For this review, use the dimensioned drawing (mm, ordinates from the lowest corner) and the shaded views. A direction names the side the tool comes from. Coordinates: 2 decimals unless noted, no trailing zeros. Write each loop counter-clockwise with the first axis right and the second up, starting at its lowest first coordinate (ties: lowest second). Pieces come first, ordered by that corner, then holes. Notation, with made-up numbers: (21.25, -8.5) -> (80.25, -8.5) arc R22 cw to (80.25, 2.5) -> close; hole circle Ø5 at (40, 12.5). An arc over 180 degrees is marked (long way). Return JSON: item names as keys, results as strings. Group by question number.
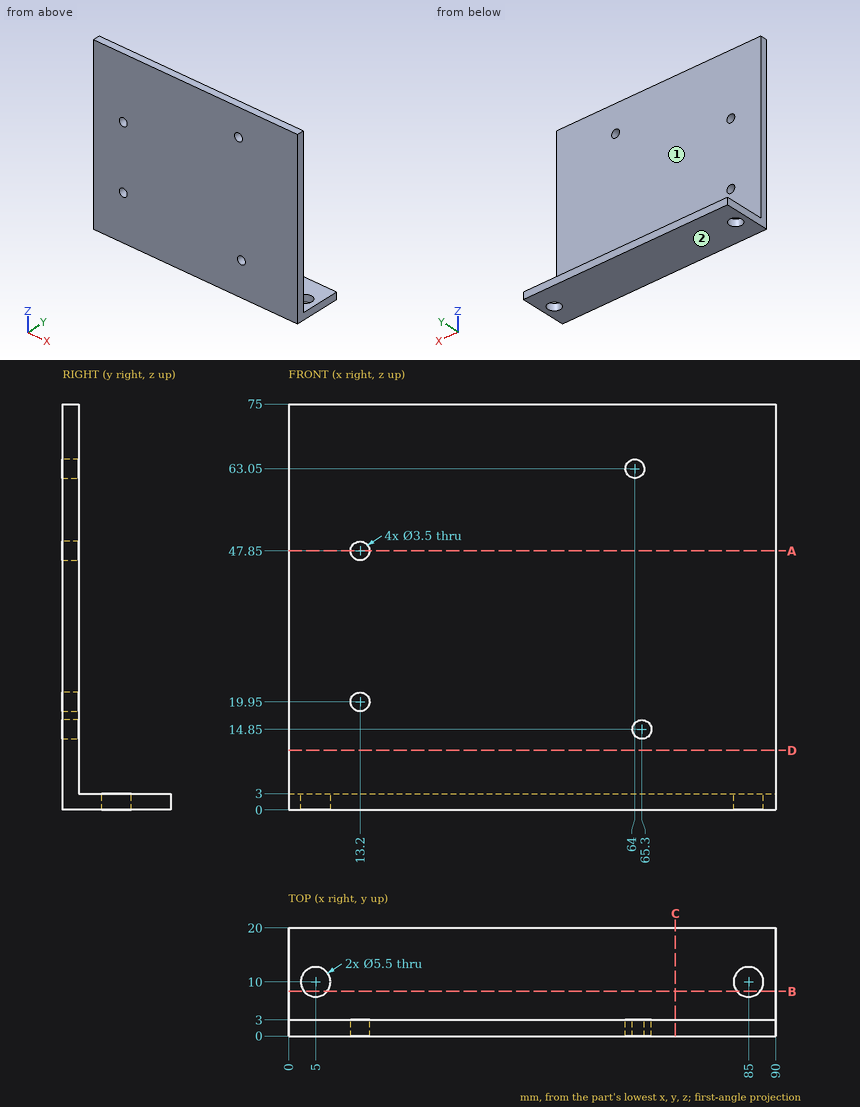
Q1. We need section A-A on z = 47.85. Write out the cut boundary in (x, y).
Q2. We need section B-B on y = 8.25. Write out the cut boundary in (x, z), plus the area to 3 significant figures.
Q3. For P1, Ø21.5, axis at x = 44.5, z = 34, coming from the +Y side; P2, Ø3.5, axis at x = 85, y = 10, coming from the -Z side; P3, Ø4, axis at x = 19.5, y = 5.5, coming from the +Z side, all flat-tipped, find the tip position at first contact; note any pin that passes through.
Q4. We need section C-C on x = 71.5. Write out the cut boundary in (y, z).
Q5. We need section D-D on z = 11. Write out the cut boundary in (x, y), plus the area to 3 significant figures.
Q6. Wall thickness on L1, parallel to X at y = 1.85, z = 14.85; L2, parallel to Z at x = 65.3, y = 2.1; L3, parallel to X at y = 1.3, z = 47.85: over which ranges is each line inside the solid? List them lowest first.
Q7. For the marked faces 1 and 2, list the 3-axis set-ups (+Z, -Z, +X, -X, +Y, -Y) from which the entire face can be reached by the end or side of a thin tool; tool diameter is ignored.
Findings below:
{
 "1": {"outline": "(0, 0) -> (11.45, 0) -> (11.45, 3) -> (0, 3) -> close; (14.95, 0) -> (90, 0) -> (90, 3) -> (14.95, 3) -> close"},
 "2": {"outline": "(0, 0) -> (2.88, 0) -> (2.88, 3) -> (0, 3) -> close; (7.12, 0) -> (82.88, 0) -> (82.88, 3) -> (7.12, 3) -> close; (87.12, 0) -> (90, 0) -> (90, 3) -> (87.12, 3) -> close", "area": "245 mm^2"},
 "3": {"P1": "stops at y = 3", "P2": "passes through", "P3": "stops at z = 3"},
 "4": {"outline": "(0, 0) -> (20, 0) -> (20, 3) -> (3, 3) -> (3, 75) -> (0, 75) -> close"},
 "5": {"outline": "(0, 0) -> (90, 0) -> (90, 3) -> (0, 3) -> close", "area": "270 mm^2"},
 "6": {"L1": "x = 0 to 63.55, 67.05 to 90", "L2": "z = 0 to 13.1, 16.6 to 61.88, 64.22 to 75", "L3": "x = 0 to 11.45, 14.95 to 90"},
 "7": {"face 1": "+Z, +X, -X, +Y", "face 2": "-Z, +X, -X, +Y, -Y"}
}
